Design review of the part built by this model. Coordinates are the model's own, in mm. A direction names the side the tool comes from. Give positions to 0.01 mm unless a question says otherwise; leave off trailing zeros. Loops run counter-clockwise (first coordinate to the right, second up) from the corner with the lowest first, then second, coordinate; pieces in that order, holes last. Notation, with made-up numbers: M 71.5,-4.75 L 103.5,-4.75 A21 cw 103.5,3.25 Z; hole C 16.5,82.25 d10. An arc over 180 degrees is marked long. Use a Markdown table: item, result. Add a question column.
(1) Add section D-D, the plane z = 7.25. Give the boundary of the cut face in (x, y).
(2) Draft analysis for pull direction Y (two halves, no side actions). For faces 1 (the face through (-7.5, 4, 35)), 2 (the face through (6.07, -5.5, 33.37)), 3 (the face through (8.75, -8.45, 43.07)), state which applies: pulls with the +Y half, pulls with the -Y half, needs draft (parallel to the pull), parting line crosses it, or undercut.
(3) For probe 1 along Y at (x, z) = (10, 42.5); probe 2 along Y at (x, z) = (10, 44.75); probe 3 along Z at (x, y) = (0, -7.6), list the stretches that pass through material, from the lowest coordinate up.
(4) For faces 4 (the face through (-10, 2, 26)), 5 (the face through (10, 7, 43)), 6 (the face through (6, -7, 17)), 7 (the face through (-17, -3, 43)), 8 (the face through (0, -8, 38)), list the 3-axis set-ups (+Z, -Z, +X, -X, +Y, -Y) from which the entire face can be reached by the end or side of a thin tool; tool diameter is ignored.
(5) Add section A-A, the plane y = 1.5. Give the boundary of the cut face in (x, z).
(6) Insertion check: pin 1 Ø1 at (x, y) = (-9.5, 7) entering from -Z; pin 2 Ø1.2 at (x, y) = (17.5, -3.5) entering from -Z; pin 3 Ø2 at (x, y) = (0, -8.5) entering from +Z. Each pin has a flat end and moves straight along its axis. Give the tip position at first contact, or say it passes through.
(7) Add section B-B, the plane z = 21.5. Give the boundary of the cut face in (x, y).
(8) Add section C-C, the plane x = 5. Give the boundary of the cut face in (y, z).
```python
from build123d import *

# Parameters (mm, degrees)
SKETCH1_W            = 25
SKETCH1_H            = 20
MAIN_DEPTH           = 43
SKETCH5_R            = 1.05
SKETCH5_R_2          = 7.15
MAINANDFIXHOLE_DEPTH = 21
SKETCH6_R            = 2.2
CODERFIXHOLE2_DEPTH  = 1.5
SKETCH7_W            = 26
SKETCH7_H            = 17
CODERHOLE_DEPTH      = 26
SKETCH10_W           = 36
SKETCH10_H           = 14
LINK_DEPTH           = 5
SKETCH8_R            = 1.25
VERTICALHOLES_DEPTH  = 10
SKETCH9_W            = 15
SKETCH9_H            = 17
CUT_EXTRUDE6_DEPTH   = 17
FILLET2_R            = 2
FILLET3_R            = 5
FILLET4_R            = 3
FILLET5_R            = 12


with BuildPart() as part:
    # Sketch1 → Main (new body)
    with BuildSketch(Plane.XY):
        Rectangle(SKETCH1_W, SKETCH1_H)
    extrude(amount=MAIN_DEPTH)

    # Sketch5 → MainAndFixHole (cut, through all)
    with BuildSketch(Plane(origin=(0, -10, 0), x_dir=(-1, 0, 0), z_dir=(0, -1, 0))):
        with Locations((0, -21.5)):
            Circle(SKETCH5_R)
        with Locations((-8.227241336, -7.25)):
            Circle(SKETCH5_R)
        with Locations((8.227241336, -7.25)):
            Circle(SKETCH5_R)
        with Locations((0, -12)):
            Circle(SKETCH5_R_2)
    extrude(amount=-MAINANDFIXHOLE_DEPTH, mode=Mode.SUBTRACT)

    # Sketch6 → CoderFixHole2 (cut)
    with BuildSketch(Plane(origin=(0, -10, 0), x_dir=(-1, 0, 0), z_dir=(0, -1, 0))):
        with Locations((0, -21.5)):
            Circle(SKETCH6_R)
        with Locations((-8.227241336, -7.25)):
            Circle(SKETCH6_R)
        with Locations((8.227241336, -7.25)):
            Circle(SKETCH6_R)
    extrude(amount=-CODERFIXHOLE2_DEPTH, mode=Mode.SUBTRACT)

    # Sketch7 → CoderHole (cut, through all)
    with BuildSketch(Plane(origin=(12.5, 0, 0), x_dir=(0, 0, -1), z_dir=(1, 0, 0))):
        with Locations((-13, 1.5)):
            Rectangle(SKETCH7_W, SKETCH7_H)
    extrude(amount=-CODERHOLE_DEPTH, mode=Mode.SUBTRACT)

    # Sketch10 → Link (add)
    with BuildSketch(Plane.XY.offset(43)):
        with Locations((0, -3)):
            Rectangle(SKETCH10_W, SKETCH10_H)
    extrude(amount=LINK_DEPTH)

    # Sketch8 → VerticalHoles (cut)
    with BuildSketch(Plane.XY.offset(48)):
        with Locations((-10, 1.5)):
            Circle(SKETCH8_R)
        with Locations((-10, -8.5)):
            Circle(SKETCH8_R)
        with Locations((10, -8.5)):
            Circle(SKETCH8_R)
        with Locations((10, 1.5)):
            Circle(SKETCH8_R)
        with Locations((-10, -3.5)):
            Circle(SKETCH8_R)
        with Locations((10, -3.5)):
            Circle(SKETCH8_R)
        with Locations((0, 1.5)):
            Circle(SKETCH8_R)
        with Locations((0, -8.5)):
            Circle(SKETCH8_R)
    extrude(amount=-VERTICALHOLES_DEPTH, mode=Mode.SUBTRACT)

    # Sketch9 → Cut-Extrude6 (cut)
    with BuildSketch(Plane(origin=(0, 10, 0), x_dir=(1, 0, 0), z_dir=(0, 1, 0))):
        with Locations((0, -34.5)):
            Rectangle(SKETCH9_W, SKETCH9_H)
    extrude(amount=-CUT_EXTRUDE6_DEPTH, mode=Mode.SUBTRACT)

    # Fillet2
    fillet2_edges = [part.edges().sort_by_distance(p)[0] for p in [
        (10, -7, 26),
        (-10, -7, 26),
    ]]
    fillet(fillet2_edges, radius=FILLET2_R)

    # Fillet3
    fillet3_edges = [part.edges().sort_by_distance(p)[0] for p in [
        (-7.5, -7, 34.5),
        (7.5, -7, 34.5),
    ]]
    fillet(fillet3_edges, radius=FILLET3_R)

    # Fillet4
    fillet4_edges = [part.edges().sort_by_distance(p)[0] for p in [
        (12.5, -3, 43),
        (-12.5, -3, 43),
    ]]
    fillet(fillet4_edges, radius=FILLET4_R)

    # Fillet5
    fillet5_edges = [part.edges().sort_by_distance(p)[0] for p in [
        (-12.5, -8.5, 0),
        (12.5, -8.5, 0),
    ]]
    fillet(fillet5_edges, radius=FILLET5_R)


solid = part.part
```
Established:
| question | item | result |
|---|---|---|
| 1 | outline | M -11.52,-10 L -10.43,-10 L -10.43,-8.5 L -9.28,-8.5 L -9.28,-7 L -11.52,-7 Z; M -7.18,-8.5 L -6.03,-8.5 L -6.03,-10 L -5.34,-10 L -5.34,-7 L -7.18,-7 Z; M 5.34,-10 L 6.03,-10 L 6.03,-8.5 L 7.18,-8.5 L 7.18,-7 L 5.34,-7 Z; M 9.28,-8.5 L 10.43,-8.5 L 10.43,-10 L 11.52,-10 L 11.52,-7 L 9.28,-7 Z |
| 2 | face 1 | needs draft |
| 2 | face 2 | pulls with the +Y half |
| 2 | face 3 | undercut |
| 3 | probe 1 | -10 to -9.75, -7.25 to -4.75, -2.25 to 0.25, 2.75 to 10 |
| 3 | probe 2 | -10 to -9.75, -7.25 to -4.75, -2.25 to 0.25, 2.75 to 4 |
| 3 | probe 3 | 0 to 4.85, 19.15 to 20.45, 22.55 to 38 |
| 4 | face 4 | -Z, +X, -X, +Y |
| 4 | face 5 | +Z, +X, -X, +Y |
| 4 | face 6 | -Z, +Y |
| 4 | face 7 | -Z, -X, +Y, -Y |
| 4 | face 8 | +Z |
| 5 | outline | M -18,43 L -15.5,43 A3 cw -12.5,40 L -12.5,26 L -7.5,26 L -7.5,43 L -1.25,43 L -1.25,48 L -8.75,48 L -8.75,38 L -11.25,38 L -11.25,48 L -18,48 Z; M 1.25,43 L 7.5,43 L 7.5,26 L 12.5,26 L 12.5,40 A3 cw 15.5,43 L 18,43 L 18,48 L 11.25,48 L 11.25,38 L 8.75,38 L 8.75,48 L 1.25,48 Z |
| 6 | pin 1 | z = 26 |
| 6 | pin 2 | z = 43 |
| 6 | pin 3 | z = 38 |
| 7 | outline | M -12.5,-10 L -2.2,-10 L -2.2,-8.5 L -1.05,-8.5 L -1.05,-7 L -12.5,-7 Z; M 1.05,-8.5 L 2.2,-8.5 L 2.2,-10 L 12.5,-10 L 12.5,-7 L 1.05,-7 Z |
| 8 | outline | M -10,0.88 L -7,0.88 L -7,6.89 L -10,6.89 Z; M -10,17.11 L -7,17.11 L -7,24 A2 cw -6.33,25.49 L -6.33,43 L 4,43 L 4,48 L -10,48 Z |
